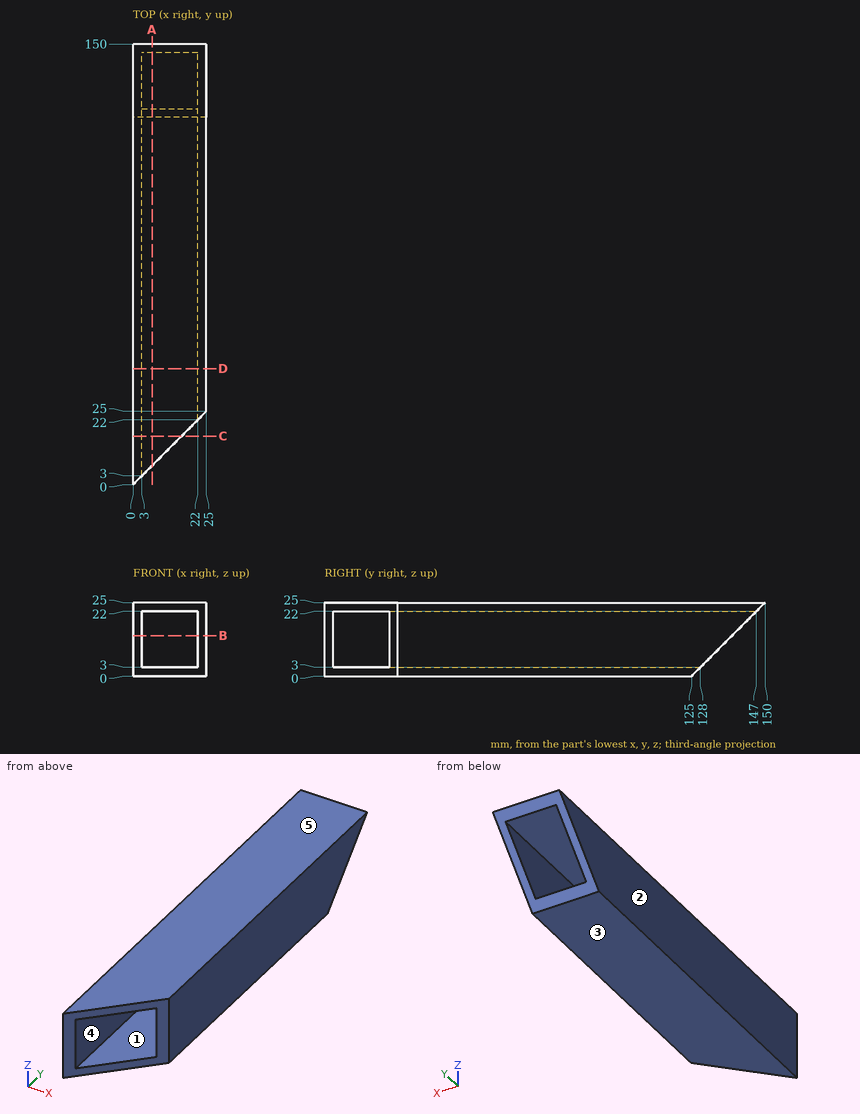
Study the drawing (mm; zero at the part's minimum x, y, z) and answer. A direction names the side the tool comes from. Coordinates: 2 decimals unless noted, no trailing zeros. Write each loop counter-clockwise with the first axis right and the second up, starting at its lowest first coordinate (ties: lowest second). Pieces come first, ordered by that corner, then holes. Notation, with made-up numbers: (77, 64.5) - (88, 64.5) arc R22 ccw to (88, 99.5) - close; hole circle Ø3 at (53.25, 66). An arc over 180 degrees is marked (long way). One line per question, with ' | ' between items.
1) Find section D-D, the plane y = 39.5. Determine the outline of the cut face in (x, z), and give its area (3 significant figures).
Checks:
outline: (0, 0) - (25, 0) - (25, 25) - (0, 25) - close; hole (3, 3) - (22, 3) - (22, 22) - (3, 22) - close | area: 264 mm2
2) Find section B-B, the plane z = 13.75. Determine the outline of the cut face in (x, y), and give its area (4 significant figures).
Checks:
outline: (0, 0) - (3, 3) - (3, 138.75) - (0, 138.75) - close; (22, 22) - (25, 25) - (25, 138.75) - (22, 138.75) - close | area: 757.5 mm2
3) Find section A-A, the plane x = 6.5. Determine the outline of the cut face in (y, z), and give its area (3 significant figures).
Checks:
outline: (6.5, 0) - (125, 0) - (128, 3) - (6.5, 3) - close; (6.5, 22) - (147, 22) - (150, 25) - (6.5, 25) - close | area: 786 mm2
4) Find section C-C, the plane y = 16.5. Determine the outline of the cut face in (x, z).
Checks:
outline: (0, 0) - (16.5, 0) - (16.5, 3) - (3, 3) - (3, 22) - (16.5, 22) - (16.5, 25) - (0, 25) - close
5) The mould has two halves that part along Z. Classify the marked faces 1, 2 and 3: +Z half, -Z half, draft (parallel to the pull), parting line (faces both ways), or undercut.
Checks:
face 1: undercut | face 2: draft | face 3: -Z half
6) Consider probe 1 along X at (y, z) = (117, 17.5); probe 2 along Y at (x, z) = (2, 2.75). Determine where each line is inside the solid, lowest interval first. Write a range as [from, to].
Checks:
probe 1: [0, 3], [22, 25] | probe 2: [2, 127.75]
7) Flat-ended cylindrical pins translate along their axes: P1, Ø1.5, axis at x = 10.5, z = 21, coming from the +Y side; P2, Ø5, axis at x = 3.5, z = 22, coming from the +Y side; P3, Ø4, axis at x = 4.5, z = 18.5, coming from the -Y side. Find the tip coordinate at first contact, or state that the pin passes through.
Checks:
P1: through | P2: y = 149.5 | P3: y = 2.5
8) For the marked faces 4 and 5, determine the directions among +Z, -Z, +X, -X, +Y, -Y from which every point of the face is accessible in a straight line to the end or side of a thin tool.
Checks:
face 4: +Y, -Y | face 5: +Z, +X, -X, +Y, -Y
